Build history of the part. All positions in model axes, mm. Coordinates: 2 decimals unless noted, no trailing zeros. Order: outer loops, then holes, each group sorted by start corner. A loop starts at its lowest first (then second) coordinate and runs counter-clockwise, first axis right, second up. Notation, with made-up numbers: (39, 14) - (60, 14) arc R23 ccw to (60, 50) - close; hole circle Ø1 at (64, 13.25). An arc over 180 degrees is marked (long way). Write each question's results on one line, items separated by ' | '. Start each with the question number.
from build123d import *

# Parameters (mm, degrees)
SKETCH1_W                 = 247.65
SKETCH1_H                 = 8
BOSS_EXTRUDE1_DEPTH       = 2
SKETCH2_W                 = 4
SKETCH2_H                 = 1
CUT_EXTRUDE1_DEPTH        = 248.65
CUT_EXTRUDE2_DEPTH        = 2.5
F_0_80_TAPPED_HOLE1_D     = 1.19126
F_0_80_TAPPED_HOLE1_DEPTH = 4.572
F_0_80_TAPPED_HOLE1_TIP   = 0.357890611


with BuildPart() as part:
    # Sketch1 → Boss-Extrude1 (new body)
    with BuildSketch(Plane(origin=(0, 0, 0), x_dir=(1, 0, 0), z_dir=(0, 1, 0))):
        Rectangle(SKETCH1_W, SKETCH1_H)
    extrude(amount=BOSS_EXTRUDE1_DEPTH)

    # Sketch2 → Cut-Extrude1 (cut, through all)
    with BuildSketch(Plane(origin=(123.825, 0, 0), x_dir=(0, 0, -1), z_dir=(1, 0, 0))):
        Rectangle(SKETCH2_W, SKETCH2_H)
    extrude(amount=-CUT_EXTRUDE1_DEPTH, mode=Mode.SUBTRACT)

    # Sketch5 → Cut-Extrude2 (cut, through all)
    with BuildSketch(Plane(origin=(0, 0.5, 0), x_dir=(-1, 0, 0), z_dir=(0, 1, 0))):
        with BuildLine():
            Line((-15.1088, -1.5), (-24.1088, -1.5))
            ThreePointArc((-24.1088, -1.5), (-25.6088, 0), (-24.1088, 1.5))
            Line((-24.1088, 1.5), (-15.1088, 1.5))
            ThreePointArc((-15.1088, 1.5), (-13.6088, 0), (-15.1088, -1.5))
        make_face()
    extrude(amount=CUT_EXTRUDE2_DEPTH, mode=Mode.SUBTRACT)

    # #0-80 Tapped Hole1
    with Locations(Plane(origin=(0, 2, 0), x_dir=(-1, 0, 0), z_dir=(0, 1, 0))):
        with Locations((114.3, 0), (-8.7588, 0), (-30.4588, 0), (-117.475, 0)):
            Hole(F_0_80_TAPPED_HOLE1_D / 2, depth=F_0_80_TAPPED_HOLE1_DEPTH)
            with Locations((0, 0, -(F_0_80_TAPPED_HOLE1_DEPTH + F_0_80_TAPPED_HOLE1_TIP / 2))):  # 118° drill point
                Cone(0, F_0_80_TAPPED_HOLE1_D / 2, F_0_80_TAPPED_HOLE1_TIP, mode=Mode.SUBTRACT)


solid = part.part
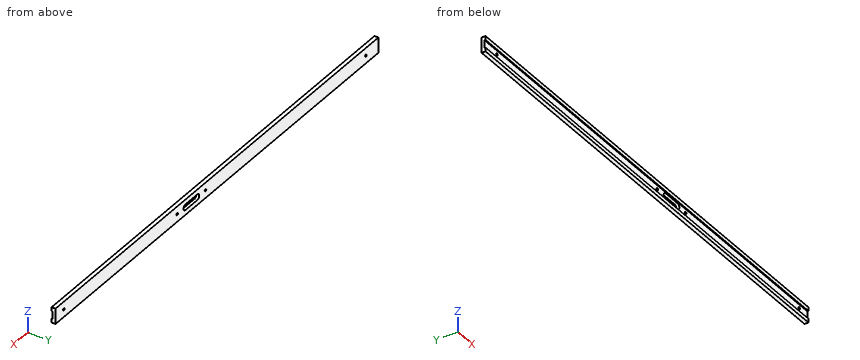
Item 1: Slice it at A-A (y = 0.8). Write the cut outline in (x, z) (3 decimals), then the cut area to 3 significant figures.
Item 2: Slice it at B-B (x = -22). Write the cut outline in (y, z).
Item 3: Flat gauge pins, fed straight in: P1, Ø1, axis at x = 77.5, z = 0.5, coming from the -Y side; P2, Ø1, axis at x = 30.46, z = 0, coming from the -Y side. Where does each tip first touch, or does it go through?
Item 4: Probe probe 1 along Z at (x, y) = (-97, 0.25); probe 2 along Y at (x, z) = (-23, -0.75); probe 3 along X at (y, z) = (1.35, 1.25) (3 decimals). List the from-to ranges inside material, lowest first.
Resolved:
1) outline: (-123.825, -4) - (123.825, -4) - (123.825, 4) - (-123.825, 4) - close; hole circle Ø1.191 at (-114.3, 0); hole circle Ø1.191 at (8.759, 0); hole (15.109, -1.5) - (24.109, -1.5) arc R1.5 ccw to (24.109, 1.5) - (15.109, 1.5) arc R1.5 ccw to start; hole circle Ø1.191 at (30.459, 0); hole circle Ø1.191 at (117.475, 0) | area: 1,940 mm^2
2) outline: (0, -4) - (2, -4) - (2, 4) - (0, 4) - (0, 2) - (0.5, 2) - (0.5, -2) - (0, -2) - close
3) P1: y = 0.5 | P2: through
4) probe 1: -4 to -2, 2 to 4 | probe 2: 0.5 to 2 | probe 3: -123.825 to 14.28, 24.938 to 123.825
